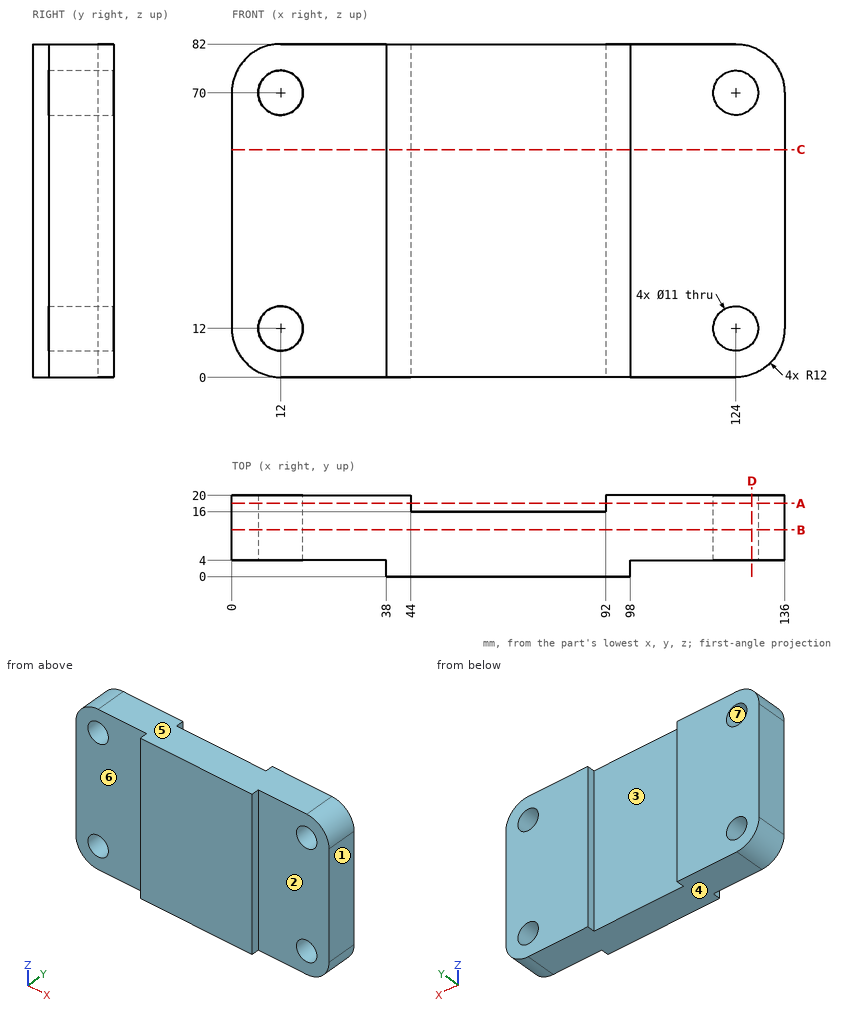
For this review, use the dimensioned drawing (mm, ordinates from the lowest corner) and the shaded views. A direction names the side the tool comes from. Give positions to 0.01 mm unless a question says otherwise; leave off trailing zeros. Order: outer loops, then holes, each group sorted by start corner. A loop starts at its lowest first (then second) coordinate and runs counter-clockwise, first axis right, second up.
1. Add section C-C, the plane z = 56. State the section outline as (x, y) points, then the cut area to 3 significant figures.
Solution:
outline: (0, 4) - (38, 4) - (38, 0) - (98, 0) - (98, 4) - (136, 4) - (136, 20) - (92, 20) - (92, 16) - (44, 16) - (44, 20) - (0, 20) - close
area: 2,220 mm2
2. Mouldability with a two-part tool opening along Z and no side actions: class the marked faces 4, 5, 6 and 7 as +Z half, -Z half, draft (parallel to the pull), parting line (faces both ways), or undercut.
Solution:
face 4: -Z half
face 5: +Z half
face 6: draft
face 7: undercut
3. Add section A-A, the plane y = 18. State the section outline as (x, z) points, then the cut area to 3 significant figures.
Solution:
outline: (0, 12) arc R12 ccw to (12, 0) - (44, 0) - (44, 82) - (12, 82) arc R12 ccw to (0, 70) - close; (92, 0) - (124, 0) arc R12 ccw to (136, 12) - (136, 70) arc R12 ccw to (124, 82) - (92, 82) - close; hole circle Ø11 at (12, 12); hole circle Ø11 at (12, 70); hole circle Ø11 at (124, 12); hole circle Ø11 at (124, 70)
area: 6,710 mm2
4. For pin 1 Ø19 at (x, z) = (114.5, 48) entering from -Y; pin 2 Ø2 at (y, z) = (1.5, 54.5) entering from -X; pin 3 Ø9 at (x, z) = (12, 12) entering from -Y; pin 4 Ø4 at (y, z) = (5, 9) entering from +X, all flat-tipped, find the tip position at first contact; note any pin that passes through.
Solution:
pin 1: stops at y = 4
pin 2: stops at x = 38
pin 3: passes through
pin 4: stops at x = 135.96
5. To check wall thickness, follow L1, parallel to Z at x = 124, y = 10.75; L2, parallel to X at y = 9, z = 70; L3, parallel to X at y = 16.25, z = 70. State the ranges of each line that lie inside material, in increasing order.
Solution:
L1: z = 0 to 6.5, 17.5 to 64.5, 75.5 to 82
L2: x = 0 to 6.5, 17.5 to 118.5, 129.5 to 136
L3: x = 0 to 6.5, 17.5 to 44, 92 to 118.5, 129.5 to 136
6. Add section B-B, the plane y = 11.5. State the section outline as (x, z) points.
Solution:
outline: (0, 12) arc R12 ccw to (12, 0) - (124, 0) arc R12 ccw to (136, 12) - (136, 70) arc R12 ccw to (124, 82) - (12, 82) arc R12 ccw to (0, 70) - close; hole circle Ø11 at (12, 12); hole circle Ø11 at (12, 70); hole circle Ø11 at (124, 12); hole circle Ø11 at (124, 70)
7. Add section D-D, the plane x = 128. State the section outline as (y, z) points, then the cut area to 3 significant figures.
Solution:
outline: (4, 0.69) - (20, 0.69) - (20, 8.23) - (4, 8.23) - close; (4, 15.77) - (20, 15.77) - (20, 66.23) - (4, 66.23) - close; (4, 73.77) - (20, 73.77) - (20, 81.31) - (4, 81.31) - close
area: 1,050 mm2
8. Tool access review of the marked faces 1, 2 and 3: name each direction out of +Z, -Z, +X, -X, +Y, -Y from which nothing blocks a thin tool from reaching the whole face with its end or side.
Solution:
face 1: +Z, -Z, +X, +Y, -Y
face 2: +Z, -Z, +X, -Y
face 3: +Z, -Z, +Y
